Can you work these out from the model? Positions are in its coordinate system, mm. Face numbers are marked on the shaded views. Give positions to 0.01 mm unless a question says otherwise; leave off trailing zeros. Order: outer loops, then holes, each group sorted by start corner. A loop starts at its lowest first (then second) coordinate and runs counter-clockwise, first axis right, second up. Notation, with made-up numbers: M 38.25,1 L 43.25,1 A33 ccw 43.25,29 Z; hole C 66,9 d11. An arc over 180 degrees is marked long. One line per question, with ' | ' between items. Start each with the question number.
1) If we section it at D-D, the plane z = -15: Please give me the cut outline in (x, y).
2) If we section it at B-B, the plane z = -27.5: Please give me the cut outline in (x, y).
3) I'm going to push flat-ended pins straight in: pin 1 Ø4 at (x, y) = (-10.5, 2.5) entering from +Z; pin 2 Ø3 at (y, z) = (6.5, -11.5) entering from -X; pin 3 Ø1.5 at (x, y) = (-10, 5.5) entering from -Z. Where does each tip first touch, or does it pass through?
4) If we section it at C-C, the plane y = 5: Please give me the cut outline in (x, z), plus the area to 3 significant figures.
5) If we section it at A-A, the plane x = 22: Please give me the cut outline in (y, z).
6) Please list where these lines run through material, in increasing order: line 1 along Z through (x, y) = (18.5, 3.5); line 2 along Z through (x, y) = (16, 2); line 3 along X through (y, z) = (2.5, -16). Write a range as [from, to].
7) Thinking about a two-plate mould opening in X: for the marked faces 1, 2 and 3, which applies, +X half, -X half, draft (parallel to the pull), parting line (faces both ways), or undercut?
```python
from build123d import *

# Parameters (mm, degrees)
BOSS_EXTRUDE1_DEPTH = 8
SKETCH2_R           = 6.85
SKETCH2_R_2         = 2.05
CUT_EXTRUDE1_DEPTH  = 8
SKETCH2_4_R         = 7.85
SKETCH2_4_R_2       = 6.85
CUT_EXTRUDE2_DEPTH  = 1.5
CUT_EXTRUDE3_START  = -6.5
SKETCH2_5_R         = 7.85
SKETCH2_5_R_2       = 6.85
SKETCH2_5_R_3       = 2.05
SKETCH2_5_R_4       = 1.4
CUT_EXTRUDE3_DEPTH  = 1.5
SKETCH2_6_R         = 1.4
CUT_EXTRUDE4_DEPTH  = 10


with BuildPart() as part:
    # Sketch1 → Boss-Extrude1 (new body)
    with BuildSketch(Plane(origin=(0, 0, 0), x_dir=(1, 0, 0), z_dir=(0, 1, 0))):
        Polygon((31.226142903, 7.08081886), (19.912434404, -4.232889639), (14.342434404, -4.232889639), (-23.841936683, 24.187416566), (-24.606695271, 29.310652291), (-23.730266729, 31.108393377), (-19.218269492, 33.568524054), (9.016403464, 28.534078393), (19.205327622, 24.661634141), (31.226142903, 12.64081886), align=None)
    extrude(amount=BOSS_EXTRUDE1_DEPTH)

    # Sketch2 → Cut-Extrude1 (cut)
    with BuildSketch(Plane(origin=(0, 8, 0), x_dir=(1, 0, 0), z_dir=(0, 1, 0))):
        with Locations(Location((17.48339004, 9.697235801, 0), (0, 0, 270))):
            Circle(SKETCH2_R)
        with Locations(Location((-18.468718365, 27.231371116, 0), (0, 0, 270))):
            Circle(SKETCH2_R_2)
    extrude(amount=-CUT_EXTRUDE1_DEPTH, mode=Mode.SUBTRACT)

    # Sketch2_4 → Cut-Extrude2 (cut)
    with BuildSketch(Plane(origin=(0, 8, 0), x_dir=(1, 0, 0), z_dir=(0, 1, 0))):
        with Locations(Location((17.48339004, 9.697235801, 0), (0, 0, 270))):
            Circle(SKETCH2_4_R)
        with Locations(Location((17.48339004, 9.697235801, 0), (0, 0, 270))):
            Circle(SKETCH2_4_R_2, mode=Mode.SUBTRACT)
    extrude(amount=-CUT_EXTRUDE2_DEPTH, mode=Mode.SUBTRACT)

    # Sketch2_5 → Cut-Extrude3 (cut)
    # profile 1 of 6: a face of its own
    with BuildSketch(Plane(origin=(0, 8, 0), x_dir=(1, 0, 0), z_dir=(0, 1, 0)).offset(CUT_EXTRUDE3_START)):
        with Locations(Location((17.48339004, 9.697235801, 0), (0, 0, 270))):
            Circle(SKETCH2_5_R)
        with Locations(Location((17.48339004, 9.697235801, 0), (0, 0, 270))):
            Circle(SKETCH2_5_R_2, mode=Mode.SUBTRACT)
    # profile 2 of 6: a face of its own
    with BuildSketch(Plane(origin=(0, 8, 0), x_dir=(1, 0, 0), z_dir=(0, 1, 0)).offset(CUT_EXTRUDE3_START)):
        with Locations(Location((-18.468718365, 27.231371116, 0), (0, 0, 270))):
            Circle(SKETCH2_5_R_3)
    # profile 3 of 6: a face of its own
    with BuildSketch(Plane(origin=(0, 8, 0), x_dir=(1, 0, 0), z_dir=(0, 1, 0)).offset(CUT_EXTRUDE3_START)):
        with Locations(Location((16.657298103, 20.980744657, 0), (0, 0, 270))):
            Circle(SKETCH2_5_R_4)
    # profile 4 of 6: a face of its own
    with BuildSketch(Plane(origin=(0, 8, 0), x_dir=(1, 0, 0), z_dir=(0, 1, 0)).offset(CUT_EXTRUDE3_START)):
        with Locations(Location((28.766898896, 10.523327737, 0), (0, 0, 90))):
            Circle(SKETCH2_5_R_4)
    # profile 5 of 6: a face of its own
    with BuildSketch(Plane(origin=(0, 8, 0), x_dir=(1, 0, 0), z_dir=(0, 1, 0)).offset(CUT_EXTRUDE3_START)):
        with Locations(Location((6.199881183, 8.871143864, 0), (0, 0, 90))):
            Circle(SKETCH2_5_R_4)
    # profile 6 of 6: a face of its own
    with BuildSketch(Plane(origin=(0, 8, 0), x_dir=(1, 0, 0), z_dir=(0, 1, 0)).offset(CUT_EXTRUDE3_START)):
        with Locations(Location((18.309481976, -1.586273056, 0), (0, 0, 270))):
            Circle(SKETCH2_5_R_4)
    extrude(amount=-CUT_EXTRUDE3_DEPTH, mode=Mode.SUBTRACT)

    # Sketch2_6 → Cut-Extrude4 (cut)
    with BuildSketch(Plane(origin=(0, 8, 0), x_dir=(1, 0, 0), z_dir=(0, 1, 0))):
        with Locations(Location((16.657298103, 20.980744657, 0), (0, 0, 270))):
            Circle(SKETCH2_6_R)
        with Locations(Location((28.766898896, 10.523327737, 0), (0, 0, 90))):
            Circle(SKETCH2_6_R)
        with Locations(Location((18.309481976, -1.586273056, 0), (0, 0, 270))):
            Circle(SKETCH2_6_R)
        with Locations(Location((6.199881183, 8.871143864, 0), (0, 0, 90))):
            Circle(SKETCH2_6_R)
    extrude(amount=-CUT_EXTRUDE4_DEPTH, mode=Mode.SUBTRACT)


solid = part.part
```
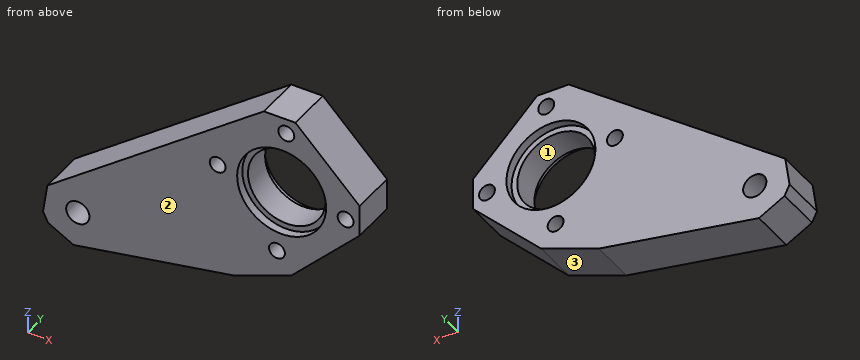
Results found:
1) outline: M -11.5,0 L 11.7,0 L 11.7,1.5 L 13.15,1.5 L 13.15,6.5 L 11.7,6.5 L 11.7,8 L -11.5,8 Z; M 21.82,1.5 L 23.27,1.5 L 23.27,0 L 28.87,0 L 28.87,8 L 23.27,8 L 23.27,6.5 L 21.82,6.5 Z
2) outline: M -24.34,0 L -20.5,0 L -20.5,8 L -24.34,8 Z; M -16.44,0 L 11.74,0 L 11.74,8 L -16.44,8 Z
3) pin 1: stops at z = -12.77 | pin 2: stops at x = -8.81 | pin 3: stops at z = -32.06
4) outline: M -24.61,-29.31 L -23.73,-31.11 L -19.22,-33.57 L 9.02,-28.53 L 19.21,-24.66 L 31.23,-12.64 L 31.23,-7.08 L 19.91,4.23 L 14.34,4.23 L -23.84,-24.19 Z; hole C -18.47,-27.23 d4.1; hole C 6.2,-8.87 d2.8; hole C 17.48,-9.7 d13.7; hole C 16.66,-20.98 d2.8; hole C 18.31,1.59 d2.8; hole C 28.77,-10.52 d2.8 | area: 965 mm²
5) outline: M 0,-21.87 L 8,-21.87 L 8,-16.12 L 6.5,-16.12 L 6.5,-14.85 L 1.5,-14.85 L 1.5,-16.12 L 0,-16.12 Z; M 0,-3.28 L 1.5,-3.28 L 1.5,-4.55 L 6.5,-4.55 L 6.5,-3.28 L 8,-3.28 L 8,2.15 L 0,2.15 Z
6) line 1: z = [-24.93, -16.47], [-2.92, 0.2], [2.97, 4.23] | line 2: z = [-25.88, -22.22], [-19.74, -16.38], [-3.01, 4.23] | line 3: x = [-12.84, 14.8], [20.17, 27.87]
7) face 1: undercut | face 2: draft | face 3: +X half
